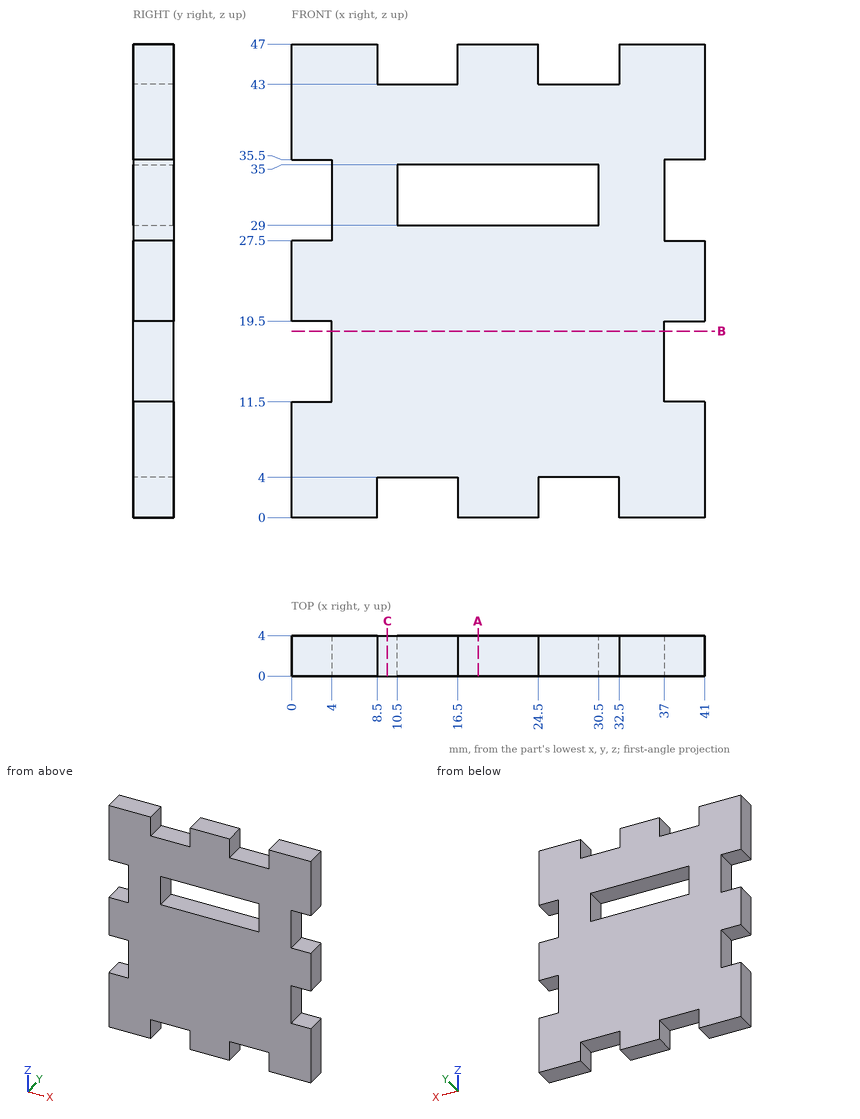
Geometry: see drawing. Coordinates: mm, zero at the bounding-box minimum. Round coordinates to 2 decimals unless told otherwise and drop trailing zeros. Order: outer loops, then holes, each group sorted by start corner. A loop starts at its lowest first (then second) coordinate and runs counter-clockwise, first axis right, second up. Notation, with made-up numbers: (5.25, -26) - (38.25, -26) arc R36 cw to (38.25, 10) - close; hole circle Ø2 at (47, 3.25). An arc over 180 degrees is marked (long way). Use a Markdown table: item, result. Add a question column.
1. Section query B-B (z = 18.5). Return the cut outline in (x, y).
2. Line query: probe 1 along Z at (x, y) = (2, 0.8); probe 2 along Z at (x, y) = (17.5, 3.5); probe 3 along Z at (x, y) = (13.5, 1.6). Output: solid intervals per line, ascending.
3. Section query A-A (x = 18.5). Return the cut outline in (y, z).
4. First-contact query: pin 1 (2 mm diameter, centred on y = 3, z = 17.5, fed in from -X); pin 2 (1 mm diameter, centred on y = 3.5, z = 15.5, fed in from +X). Flat tips, straight axial feed; report the tip coordinate or a pass-through.
5. Section query C-C (x = 9.5). Return the cut outline in (y, z), then the cut area to 3 significant figures.
Derived:
| question | item | result |
|---|---|---|
| 1 | outline | (4, 0) - (37, 0) - (37, 4) - (4, 4) - close |
| 2 | probe 1 | 0 to 11.5, 19.5 to 27.5, 35.5 to 47 |
| 2 | probe 2 | 0 to 29, 35 to 47 |
| 2 | probe 3 | 4 to 29, 35 to 43 |
| 3 | outline | (0, 0) - (4, 0) - (4, 29) - (0, 29) - close; (0, 35) - (4, 35) - (4, 47) - (0, 47) - close |
| 4 | pin 1 | x = 4 |
| 4 | pin 2 | x = 37 |
| 5 | outline | (0, 4) - (4, 4) - (4, 43) - (0, 43) - close |
| 5 | area | 156 mm2 |
